```python
from build123d import *

# Parameters (mm, degrees)
F0_W          = 35
F0_H          = 57
F1_DEPTH      = 31.5
F4_DEPTH      = 57.001
F5_DEPTH      = 35.0010001
F7_DEPTH      = 35.0010001
F9_DEPTH      = 2
F9_DEPTH_BACK = 37
F11_DEPTH     = 37.001
F12_DEPTH     = 47
F13_W         = 15
F13_H         = 4
F14_DEPTH     = 2
F15_T1_DEPTH  = 35
F16_W         = 11
F16_H         = 1
F17_DEPTH     = 1


# Not quite as in the source:
# - a fillet or chamfer that OpenCascade refuses, or shapes differently, is made with other operations: its cross-section is extruded or revolved along the edge and cut away or added


with BuildPart() as f1:
    # F0 (on Top) → F1 (new body)
    with BuildSketch(Plane.XY):
        with Locations((0.0945744105, -24.8016776452)):
            Rectangle(F0_W, F0_H)
    extrude(amount=F1_DEPTH)

    # F3 (on face) → F4 (cut, through all)
    with BuildSketch(Plane.XZ.offset(53.3016776452)):
        with BuildLine():
            add(Edge.make_bspline(
                [(0.0945744105, 2), (14.3839935729, 2), (7.2392839917, 17), (0.0945744105, 32), (-7.0501351708, 17), (-14.194844752, 2), (0.0945744105, 2)],
                knots=[0, 0, 0, 2.0943951024, 2.0943951024, 4.1887902048, 4.1887902048, 6.2831853072, 6.2831853072, 6.2831853072], degree=2, weights=[1, 0.5, 1, 0.5, 1, 0.5, 1]))
        make_face()
    extrude(amount=-F4_DEPTH, mode=Mode.SUBTRACT)

    # F2 (on face) → F5 (cut, through all)
    with BuildSketch(Plane.YZ.offset(17.5945744105)):
        with BuildLine():
            ThreePointArc((-53.3016776452, 0), (-35.9248296563, 21.279893434), (-10.4231016291, 31.5))
            Line((-10.4231016291, 31.5), (-53.3016776452, 31.5))
            Line((-53.3016776452, 31.5), (-53.3016776452, 0))
        make_face()
    extrude(amount=-F5_DEPTH, mode=Mode.SUBTRACT)

    # F6 (on face) → F7 (cut, through all)
    with BuildSketch(Plane.YZ.offset(17.5945744105)):
        with BuildLine():
            Line((3.6983223548, 0), (3.6983223548, 29))
            ThreePointArc((3.6983223548, 29), (-28.0042777095, 22.8678173622), (-50.8016776452, 0))
            Line((-50.8016776452, 0), (3.6983223548, 0))
        make_face()
    extrude(amount=-F7_DEPTH, mode=Mode.SUBTRACT)

    # F8 (on face) → F9 (join, two sides)
    with BuildSketch(Plane.YZ.offset(17.5945744105)) as f9_sk:
        with BuildLine():
            ThreePointArc((-49.9582016017, 1.5371667936), (-51.6783665277, 1.4810577961), (-50.8016776452, 0))
            ThreePointArc((-50.8016776452, 0), (-50.3860655446, 0.7719448198), (-49.9582016017, 1.5371667936))
        make_face()
        with BuildLine():
            ThreePointArc((-49.9582016017, 1.5371667936), (-50.3860655446, 0.7719448198), (-50.8016776452, 0))
            ThreePointArc((-50.8016776452, 0), (-50.094570864, 0.2928932188), (-49.8016776452, 1))
            ThreePointArc((-49.8016776452, 1), (-49.8416057615, 1.2797534241), (-49.9582016017, 1.5371667936))
        make_face()
    extrude(amount=F9_DEPTH)
    extrude(f9_sk.sketch, amount=-F9_DEPTH_BACK)

    # F10 (on face) → F11 (cut, through all)
    with BuildSketch(Plane.YZ.offset(17.5945744105)):
        with BuildLine():
            Line((-53.3016776452, 0), (-52.3163572735, 0))
            ThreePointArc((-52.3163572735, 0), (-52.6137174082, 0.8962393447), (-52.4206060402, 1.8205639696))
            ThreePointArc((-52.4206060402, 1.8205639696), (-52.8695111773, 0.9143323688), (-53.3016776452, 0))
        make_face()
    extrude(amount=-F11_DEPTH, mode=Mode.SUBTRACT)

    # F12 (add): a face of the model
    f12_faces = [f1.faces().sort_by_distance(p)[0] for p in [
        (0.0945744105, 3.6983223548, 30.25),
    ]]
    extrude(f12_faces, amount=F12_DEPTH)

    # F13 (on face) → F14 (join)
    with BuildSketch(Plane.XY.offset(31.5)):
        with Locations((0.0945744105, 48.6983223548)):
            Rectangle(F13_W, F13_H)
    extrude(amount=F14_DEPTH)

    # F15: fillet of radius 5 on 1 edges, made by hand

    # F15_s2 → F15_t1 (cut)
    with BuildSketch(Plane.YZ.offset(-17.4054255895)):
        with BuildLine():
            ThreePointArc((46.6983223548, 31.5), (48.4622543773, 32.972135955), (50.6983223548, 33.5))
            Line((50.6983223548, 33.5), (46.6983223548, 33.5))
            Line((46.6983223548, 33.5), (46.6983223548, 31.5))
        make_face()
    extrude(amount=F15_T1_DEPTH, mode=Mode.SUBTRACT)

    # F16 (on face) → F17 (cut)
    with BuildSketch(Plane(origin=(0, 50.6983223548, 0), x_dir=(-1, 0, 0), z_dir=(0, 1, 0))):
        with Locations((-0.0945744105, 32.5)):
            Rectangle(F16_W, F16_H)
    extrude(amount=-F17_DEPTH, mode=Mode.SUBTRACT)


solid = f1.part
```
For this review, take the finished solid that the model builds, in its own axes (mm). A direction names the side the tool comes from. Round coordinates to 2 decimals unless told otherwise and drop trailing zeros. Write each loop counter-clockwise with the first axis right and the second up, starting at its lowest first coordinate (ties: lowest second). Pieces come first, ordered by that corner, then holes. Notation, with made-up numbers: M 84.5,72.5 L 116.5,72.5 A23 cw 116.5,85.5 Z; hole C -12.75,48 d6. An arc over 180 degrees is marked long. One line per item, written item: value. Start each with the question number.
(1) We need section A-A (x = 13). Give the boundary of the cut face in (y, z) (3 decimals).
(2) We need section B-B (y = 43). Give the boundary of the cut face in (x, z), and give its area (3 significant figures).
(3) Machinability: for faces 4 (the flat face through (7.595, 49, 32)), 5 (the flat face through (-7.405, 49, 32)), 6 (the flat face through (19.595, -51, 1)), 7 (the flat face through (0, 27, 29)), 8 (the flat face through (0, 50.698, 31)), which of the approach directions +Z, -Z, +X, -X, +Y, -Y give a long, thin tool a straight path to every point of the face, cutting with its end or side? Answer none if there is none.
(4) Insertion check: pin 1 (1.5 mm diameter, centred on y = -25.5, z = 25.5, fed in from +X); pin 2 (0.5 mm diameter, centred on x = -1.5, z = 32.5, fed in from +Y); pin 3 (6 mm diameter, centred on x = 2.5, z = 9.5, fed in from +Y); pin 4 (6 mm diameter, centred on x = 14, z = 17.5, fed in from -Y). Each pin has a flat end and moves straight along its axis. Give the tip position at first contact, or say it passes through.
(5) Wall thickness on line 1 (Z direction, x = -5, y = 46); line 2 (Y direction, x = -13, z = 23); line 3 (Z direction, x = 14, y = -13): over which ranges is each line inside the solid? List them lowest first.
(6) We need section C-C (y = -1). Give the boundary of the cut face in (x, z), and give its area (3 significant figures).
(7) The part is to be moulded in two halves that separate along Y. For faces 1 (the cylindrical face through (0.34, -20.306, 26.237)), 2 (the flat face through (0, 20, 31.5)), 3 (the cylindrical face through (0.34, -52.613, 0.883)), say which applies: released by +Y, released by -Y, zero draft, split by the parting line, or undercut.
Result:
1. outline: M -52.421,1.821 A1.815 ccw -52.316,0 L -50.802,0 A1 ccw -49.958,1.537 A55 cw 3.698,29 L 50.698,29 L 50.698,31.5 L -10.423,31.5 A55 ccw Z
2. outline: M -17.41,29 L 17.59,29 L 17.59,31.5 L -17.41,31.5 Z
2. area: 87.5 mm²
3. face 4: +Z, +X, +Y, -Y
3. face 5: +Z, -X, +Y, -Y
3. face 6: +Z, -Z, +X, +Y, -Y
3. face 7: -Z, +X, -X, +Y
3. face 8: +Z, -Z, +X, -X, +Y
4. pin 1: x = 17.59
4. pin 2: y = 49.7
4. pin 3: through
4. pin 4: y = -43.55
5. line 1: 29 to 31.5
5. line 2: -33.44 to -27.75
5. line 3: 28.24 to 31.1
6. outline: M -17.41,29.3 L 17.59,29.3 L 17.59,31.5 L -17.41,31.5 Z
6. area: 77.0 mm²
7. face 1: undercut
7. face 2: zero draft
7. face 3: released by -Y
